Verification items for the finished model (mm, model axes). A direction names the side the tool comes from. Coordinates: 2 decimals unless noted, no trailing zeros. Loops run counter-clockwise (first coordinate to the right, second up) from the corner with the lowest first, then second, coordinate; pieces in that order, holes last. Notation, with made-up numbers: (26, -18) - (77, -18) arc R9 ccw to (77, -10) - close; hole circle Ø8 at (-30, 70.5). An arc over 180 degrees is marked (long way). Answer as CSV lines item,"result". Start each with the question number.
1. Cross-section at B-B (x = -40). Enter the section's corners in (y, z).
2. Gauge pin test, flat ends, axial feed: P1, Ø13.5, axis at x = -5.5, z = 0, coming from the -Y side; P2, Ø4.5, axis at x = 4, y = 3, coming from the -Z side; P3, Ø4, axis at y = 29.5, z = -10.5, coming from the -X side; P4, Ø2, axis at x = 9, y = 2, coming from the +Z side. Record the tip position at first contact, or that the pin passes through.
3. Material ranges on line 1 (X direction, y = 1.75, z = 0); line 2 (X direction, y = 61.3, z = 0); line 3 (X direction, y = 16, z = 5.75), recorded low to high. Write a range as [from, to].
4. Release check for a two-part mould opening along X. For faces 4 (the cylindrical face through (-13.9, 1.97, -14.14)), 5 (the flat face through (-32, 33, 0)), 6 (the flat face through (45, 31, 0)) record: pulls with the +X half, pulls with the -X half, needs draft (parallel to the pull), parting line crosses it, or undercut.
5. Cross-section at C-C (x = -5.5). Enter the section's corners in (y, z).
6. Set-up check for faces 1 (the flat face through (-28, 31, 0)), 2 (the cylindrical face through (-13.9, 1.97, 14.14)), 3 (the flat face through (22, 62, -5)): record each of +Z, -Z, +X, -X, +Y, -Y from which the full face is reachable in a straight line by a thin tool's end or side.
7. Cross-section at D-D (y = 52.5). Enter the section's corners in (x, z), plus the area to 3 significant figures.
8. Cross-section at A-A (z = 0). State how many separate pieces and enclosed holes the cut face has, plus the area to 3 significant figures.
```python
from build123d import *

# Parameters (mm, degrees)
SKETCH_1_W          = 90
SKETCH_1_H          = 30
SKETCH_1_R          = 1.7
EXTRUDE_1_DEPTH     = 4
SKETCH_2_W          = 4
SKETCH_2_H          = 30
EXTRUDE_2_DEPTH     = 55
SKETCH_3_W          = 77
SKETCH_3_H          = 30
SKETCH_3_R          = 11.1
EXTRUDE_3_DEPTH     = 4
SKETCH_4_R          = 8.1
CUT_EXTRUDE_1_DEPTH = 4
SKETCH_5_W          = 21
SKETCH_5_H          = 21
CUT_EXTRUDE_2_DEPTH = 1
SKETCH_6_R          = 1.7
CUT_EXTRUDE_3_DEPTH = 5
SKETCH_7_W          = 41
SKETCH_7_H          = 7
CUT_EXTRUDE_4_DEPTH = 10
FILLET_1_R          = 3


with BuildPart() as part:
    # 草图1 → 凸台-拉伸1 (new body)
    with BuildSketch(Plane(origin=(0, 0, 0), x_dir=(1, 0, 0), z_dir=(0, 1, 0))):
        Rectangle(SKETCH_1_W, SKETCH_1_H)
        with Locations(Location((-40, 0, 0), (0, 0, 270))):
            Circle(SKETCH_1_R, mode=Mode.SUBTRACT)
    extrude(amount=EXTRUDE_1_DEPTH)

    # 草图2 → 凸台-拉伸2 (add)
    with BuildSketch(Plane(origin=(0, 4, 0), x_dir=(1, 0, 0), z_dir=(0, 1, 0))):
        with Locations((-30, 0)):
            Rectangle(SKETCH_2_W, SKETCH_2_H)
        with Locations((43, 0)):
            Rectangle(SKETCH_2_W, SKETCH_2_H)
    extrude(amount=EXTRUDE_2_DEPTH)

    # 草图3 → 凸台-拉伸3 (add)
    with BuildSketch(Plane(origin=(0, 59, 0), x_dir=(1, 0, 0), z_dir=(0, 1, 0))):
        with Locations((6.5, 0)):
            Rectangle(SKETCH_3_W, SKETCH_3_H)
        with Locations(Location((-5.5, 0, 0), (0, 0, 270))):
            Circle(SKETCH_3_R, mode=Mode.SUBTRACT)
    extrude(amount=EXTRUDE_3_DEPTH)

    # 草图4 → 切除-拉伸1 (cut)
    with BuildSketch(Plane(origin=(0, 63, 0), x_dir=(1, 0, 0), z_dir=(0, 1, 0))):
        with Locations(Location((29, 0, 0), (0, 0, 270))):
            Circle(SKETCH_4_R)
    extrude(amount=-CUT_EXTRUDE_1_DEPTH, mode=Mode.SUBTRACT)

    # 草图5 → 切除-拉伸2 (cut)
    with BuildSketch(Plane(origin=(0, 63, 0), x_dir=(1, 0, 0), z_dir=(0, 1, 0))):
        with Locations((29, 0)):
            Rectangle(SKETCH_5_W, SKETCH_5_H)
    extrude(amount=-CUT_EXTRUDE_2_DEPTH, mode=Mode.SUBTRACT)

    # 草图6 → 切除-拉伸3 (cut)
    with BuildSketch(Plane(origin=(0, 4, 0), x_dir=(1, 0, 0), z_dir=(0, 1, 0))):
        with Locations(Location((18, 0, 0), (0, 0, 270))):
            Circle(SKETCH_6_R)
    extrude(amount=-CUT_EXTRUDE_3_DEPTH, mode=Mode.SUBTRACT)

    # 草图7 → 切除-拉伸4 (cut)
    with BuildSketch(Plane(origin=(0, 4, 0), x_dir=(1, 0, 0), z_dir=(0, 1, 0))):
        with Locations((7.5, -11.5)):
            Rectangle(SKETCH_7_W, SKETCH_7_H)
        with Locations((7.5, 11.5)):
            Rectangle(SKETCH_7_W, SKETCH_7_H)
    extrude(amount=-CUT_EXTRUDE_4_DEPTH, mode=Mode.SUBTRACT)

    # 圆角1
    fillet_1_edges = [part.edges().sort_by_distance(p)[0] for p in [
        (28, 2, -8),
        (-13, 2, -8),
        (-45, 2, 15),
        (-45, 2, -15),
        (28, 2, 15),
        (-13, 2, 15),
        (-13, 2, -15),
        (28, 2, -15),
        (-13, 2, 8),
        (28, 2, 8),
    ]]
    fillet(fillet_1_edges, radius=FILLET_1_R)


solid = part.part
```
Values follow:
1,outline,"(0, -15) - (4, -15) - (4, -1.7) - (0, -1.7) - close; (0, 1.7) - (4, 1.7) - (4, 15) - (0, 15) - close"
2,P1,"stops at y = 0"
2,P2,"stops at z = -8"
2,P3,"stops at x = -32"
2,P4,"stops at z = 8"
3,line 1,"x = [-45, -41.7], [-38.3, 16.3], [19.7, 45]"
3,line 2,"x = [-32, -16.6], [5.6, 20.9], [37.1, 45]"
3,line 3,"x = [-32, -28], [41, 45]"
4,face 4,"undercut"
4,face 5,"pulls with the -X half"
4,face 6,"pulls with the +X half"
5,outline,"(0, -8) - (4, -8) - (4, 8) - (0, 8) - close; (59, -15) - (63, -15) - (63, -11.1) - (59, -11.1) - close; (59, 11.1) - (63, 11.1) - (63, 15) - (59, 15) - close"
6,face 1,"+Z, -Z"
6,face 2,"+Z, -Y"
6,face 3,"+Y"
7,outline,"(-32, -15) - (-28, -15) - (-28, 15) - (-32, 15) - close; (41, -15) - (45, -15) - (45, 15) - (41, 15) - close"
7,area,"240 mm²"
8,separate pieces,"4"
8,enclosed holes,"0"
8,area,"922 mm²"
